Part model, mm, in its own coordinate system. Face numbers are marked on the shaded views. Give positions to 0.01 mm unless a question says otherwise; leave off trailing zeros. Loops run counter-clockwise (first coordinate to the right, second up) from the corner with the lowest first, then second, coordinate; pieces in that order, holes last. Notation, with made-up numbers: M 20,24.5 L 71,24.5 A15 ccw 71,53.5 Z; hole C 43.25,34 d7. An arc over 180 degrees is marked long. Answer in a Markdown table with one row per item.
from build123d import *

# Parameters (mm, degrees)
SKETCH2_W           = 38.1
SKETCH2_H           = 15.24
SKETCH2_R           = 1.5875
BOSS_EXTRUDE1_DEPTH = 2.54
SKETCH3_R           = 1.905
BOSS_EXTRUDE2_DEPTH = 10.16


with BuildPart() as part:
    # Sketch2 → Boss-Extrude1 (new body)
    with BuildSketch(Plane(origin=(0, 0, 0), x_dir=(1, 0, 0), z_dir=(0, 1, 0))):
        Rectangle(SKETCH2_W, SKETCH2_H)
        with Locations(Location((12.7, 0, 0), (0, 0, 270))):
            Circle(SKETCH2_R, mode=Mode.SUBTRACT)
        with Locations(Location((-12.7, 0, 0), (0, 0, 90))):
            Circle(SKETCH2_R, mode=Mode.SUBTRACT)
    extrude(amount=BOSS_EXTRUDE1_DEPTH)

    # Sketch3 → Boss-Extrude2 (add)
    with BuildSketch(Plane.XZ):
        with Locations(Location((0, 0, 0), (0, 0, 270))):
            Circle(SKETCH3_R)
    extrude(amount=BOSS_EXTRUDE2_DEPTH)


solid = part.part
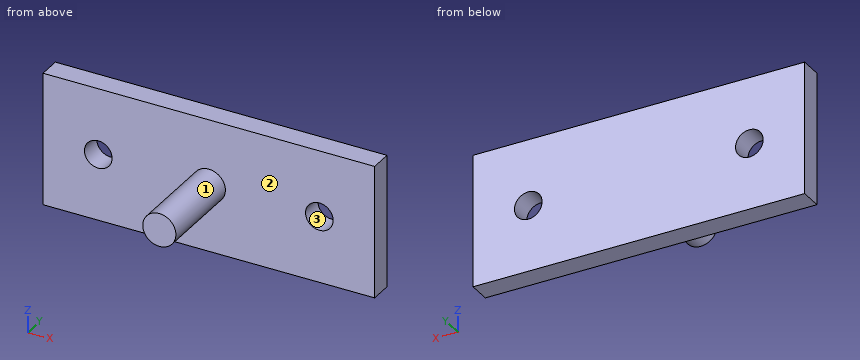
(1) Drill centre lines: line 1 along X through (y, z) = (0.95, 0); line 2 along Z through (x, y) = (-12.7, 1.7); line 3 along Y through (x, z) = (7, -4). Where is each one in solid material? Low to high.
Recorded:
| item | result |
|---|---|
| line 1 | x = -19.05 to -14.29, -11.11 to 11.11, 14.29 to 19.05 |
| line 2 | z = -7.62 to -1.59, 1.59 to 7.62 |
| line 3 | y = 0 to 2.54 |
(2) Saw through at D-D (x = 0). Write the cut outline in (y, z) (3 decimals), plus the area to 3 significant figures.
Recorded:
| item | result |
|---|---|
| outline | M -10.16,-1.905 L 0,-1.905 L 0,-7.62 L 2.54,-7.62 L 2.54,7.62 L 0,7.62 L 0,1.905 L -10.16,1.905 Z |
| area | 77.4 mm^2 |
(3) Pin check, flat tips, straight feed: pin 1 Ø2 at (x, y) = (1, -1.5) entering from +Z (3 decimals); pin 2 Ø1.5 at (x, y) = (-12, -1.5) entering from -Z; pin 3 Ø4 at (x, z) = (-12.7, 0) entering from -Y. Stop position of each tip, or through.
Recorded:
| item | result |
|---|---|
| pin 1 | stops at z = 1.905 |
| pin 2 | passes through |
| pin 3 | stops at y = 0 |
(4) Saw through at A-A (z = 0). Give the number of separate pieces and of enclosed holes in the cut face, plus the area to 3 significant figures.
Recorded:
| item | result |
|---|---|
| separate pieces | 3 |
| enclosed holes | 0 |
| area | 119 mm^2 |
(5) Saw through at B-B (x = 12.7). Write the cut outline in (y, z).
Recorded:
| item | result |
|---|---|
| outline | M 0,-7.62 L 2.54,-7.62 L 2.54,-1.59 L 0,-1.59 Z; M 0,1.59 L 2.54,1.59 L 2.54,7.62 L 0,7.62 Z |
(6) Pull direction Z, two halves, no side cores. Call the marked faces 1, 2 and 3: +Z half, -Z half, draft (parallel to the pull), parting line (faces both ways), or undercut.
Recorded:
| item | result |
|---|---|
| face 1 | parting line |
| face 2 | draft |
| face 3 | undercut |
